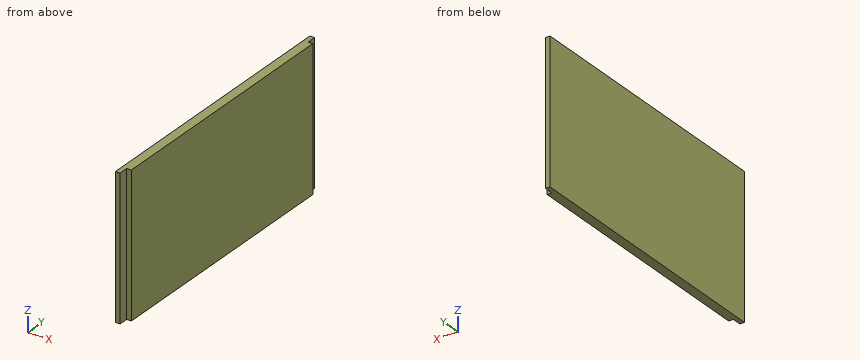
from build123d import *

# Parameters (mm, degrees)
F1_DEPTH = 150
F4_DEPTH = 150


with BuildPart() as f1:
    # F0 (on Top) → F1 (new body)
    with BuildSketch(Plane.XY):
        Polygon((0, 75), (-6, 75), (-6, -75), (0, -75), (0, -63), (6, -63), (6, 63), (0, 63), align=None)
    extrude(amount=F1_DEPTH)


with BuildPart() as f4:
    # F3 (on Top) → F4 (new body)
    with BuildSketch(Plane.XY):
        Polygon((0, 140), (0, 150), (-5, 150), (-5, -150), (0, -150), (0, -140), (5, -140), (5, 140), align=None)
    extrude(amount=F4_DEPTH)


solid = f4.part
Verification items for the finished model (mm, model axes). Give positions to 0.01 mm unless a question says otherwise; leave off trailing zeros. Loops run counter-clockwise (first coordinate to the right, second up) from the corner with the lowest first, then second, coordinate; pieces in that order, holes last.
1) Sectioned sample at B-B, the plane x = 2. Enter the section's corners in (y, z).
2) Depth check by flat-ended pin: pin 1 Ø3 at (x, z) = (2.5, 115.5) entering from -Y; pin 2 Ø4 at (x, z) = (1.5, 78.5) entering from +Y; pin 3 Ø8 at (y, z) = (145, 97.5) entering from +X. Enter the tip coordinate at first touch or a pass-through.
3) Thickness scan on line 1 along Y through (x, z) = (2.75, 134). Record the ranges inside material, lowest first.
4) Sectioned sample at A-A, the plane z = 80.5. Enter the section's corners in (x, y), then the cut area to 3 significant figures.
Answers:
1. outline: (-140, 0) - (140, 0) - (140, 150) - (-140, 150) - close
2. pin 1: stops at y = -140
2. pin 2: stops at y = 150
2. pin 3: stops at x = 0
3. line 1: y = -140 to 140
4. outline: (-5, -150) - (0, -150) - (0, -140) - (5, -140) - (5, 140) - (0, 140) - (0, 150) - (-5, 150) - close
4. area: 2,900 mm2
